Build history of the part. All positions in model axes, mm. A direction names the side the tool comes from. Round coordinates to 2 decimals unless told otherwise and drop trailing zeros. Loops run counter-clockwise (first coordinate to the right, second up) from the corner with the lowest first, then second, coordinate; pieces in that order, holes last. Notation, with made-up numbers: (45, 19) - (63, 19) arc R27 ccw to (63, 50) - close; hole circle Ø4 at (83.25, -23). An arc over 180 degrees is marked (long way). Use one line per item in the form item = value. Start each with the question number.
Q1. Saw through at D-D (x = 57.5). Give the cut face in (y, z) (3 decimals).
Q2. Pin check, flat tips, straight feed: pin 1 (1 mm diameter, centred on x = 14, z = 2, fed in from -Y); pin 2 (1 mm diameter, centred on x = 37, y = 2.5, fed in from -Z). Stop position of each tip, or through.
Q3. Saw through at B-B (x = 38.1). Give the cut face in (y, z) (3 decimals).
Q4. Saw through at A-A (y = 2.54). Give the cut face in (x, z) (3 decimals).
Q5. Mould opens along X. For faces 4 (the face through (37, 6, 3.175)), 5 (the face through (57, 5.08, 2)) say: released by +X, released by -X, zero draft, split by the parting line, or undercut.
Q6. 3-axis set-ups, long thin cutter, end or side, ignore diameter. For faces 1 (the face through (4.656, -0.215, 1.61)), 2 (the face through (71.571, 5.307, 1.61)), 3 (the face through (-0.55, 0.06, 1.57)): which of +Z, -Z, +X, -X, +Y, -Y reach the whole face in a straight line?
Q7. Saw through at C-C (z = 1.9). Give the cut face in (x, y).
Q8. Drill centre lines: line 1 (X direction, y = 2.54, z = 0.7); line 2 (Y direction, x = 76, z = 0.8); line 3 (X direction, y = 0.75, z = 0.4). Where is each one in solid material? Low to high.
```python
from build123d import *

# Parameters (mm, degrees)
SKETCH1_R               = 5.08
SKETCH1_W               = 76.2
SKETCH1_H               = 5.08
BOSS_EXTRUDE1_DEPTH     = 3.175
CUT_EXTRUDE1_DEPTH      = 82.698123754
CUT_EXTRUDE1_DEPTH_BACK = 82.698123754
SKETCH2_R               = 2.54
FILLET1_R               = 2.54


with BuildPart() as part:
    # Sketch1 → Boss-Extrude1 (new body)
    with BuildSketch(Plane.XY):
        with Locations((0, 2.54)):
            Circle(SKETCH1_R)
        with Locations((76.2, 2.54)):
            Circle(SKETCH1_R)
        with Locations((38.1, 2.54)):
            Circle(SKETCH1_R)
        with Locations((38.1, 2.54)):
            Rectangle(SKETCH1_W, SKETCH1_H)
    extrude(amount=BOSS_EXTRUDE1_DEPTH)

    # Sketch2 → Cut-Extrude1 (cut, two sides: drawn at the far end of the back side and taken through both)
    with BuildSketch(Plane.XY.offset(3.175).offset(-CUT_EXTRUDE1_DEPTH_BACK)):
        with Locations((0, 2.54)):
            Circle(SKETCH2_R)
        with Locations((76.2, 2.54)):
            Circle(SKETCH2_R)
        with Locations((38.1, 2.54)):
            Circle(SKETCH2_R)
    extrude(amount=CUT_EXTRUDE1_DEPTH + CUT_EXTRUDE1_DEPTH_BACK, mode=Mode.SUBTRACT)

    # Fillet1
    fillet1_edges = [part.edges().sort_by_distance(p)[0] for p in [
        (4.399409051, 5.08, 1.5875),
        (33.700590949, 5.08, 1.5875),
        (42.499409051, 5.08, 1.5875),
        (71.800590949, 5.08, 1.5875),
        (71.800590949, 0, 1.5875),
        (4.399409051, 0, 1.5875),
        (33.700590949, 0, 1.5875),
        (42.499409051, 0, 1.5875),
    ]]
    fillet(fillet1_edges, radius=FILLET1_R)


solid = part.part
```
Report:
q1.outline = (0, 0) - (5.08, 0) - (5.08, 3.175) - (0, 3.175) - close
q2.pin_1 = 0
q2.pin_2 = through
q3.outline = (-2.54, 0) - (0, 0) - (0, 3.175) - (-2.54, 3.175) - close; (5.08, 0) - (7.62, 0) - (7.62, 3.175) - (5.08, 3.175) - close
q4.outline = (-5.08, 0) - (-2.54, 0) - (-2.54, 3.175) - (-5.08, 3.175) - close; (2.54, 0) - (35.56, 0) - (35.56, 3.175) - (2.54, 3.175) - close; (40.64, 0) - (73.66, 0) - (73.66, 3.175) - (40.64, 3.175) - close; (78.74, 0) - (81.28, 0) - (81.28, 3.175) - (78.74, 3.175) - close
q5.face_4 = zero draft
q5.face_5 = undercut
q6.face_1 = +Z, -Z, -Y
q6.face_2 = +Z, -Z, +Y
q6.face_3 = +Z, -Z
q7.outline = (3.79, -0.85) arc R2.54 cw to (5.68, 0) - (32.42, 0) arc R2.54 cw to (34.31, -0.85) arc R5.08 ccw to (41.89, -0.85) arc R2.54 cw to (43.78, 0) - (70.52, 0) arc R2.54 cw to (72.41, -0.85) arc R5.08 ccw (long way) to (72.41, 5.93) arc R2.54 cw to (70.52, 5.08) - (43.78, 5.08) arc R2.54 cw to (41.89, 5.93) arc R5.08 ccw to (34.31, 5.93) arc R2.54 cw to (32.42, 5.08) - (5.68, 5.08) arc R2.54 cw to (3.79, 5.93) arc R5.08 ccw (long way) to start; hole circle Ø5.08 at (0, 2.54); hole circle Ø5.08 at (38.1, 2.54); hole circle Ø5.08 at (76.2, 2.54)
q8.line_1 = -5.08 to -2.54, 2.54 to 35.56, 40.64 to 73.66, 78.74 to 81.28
q8.line_2 = -2.54 to 0.01, 5.07 to 7.62
q8.line_3 = -4.75 to -1.8, 1.8 to 36.3, 39.9 to 74.4, 78 to 80.95
